from build123d import *

# Parameters (mm, degrees)
F0_W     = 76.2
F0_H     = 50.8
F0_R     = 12.7
F1_DEPTH = 12.7
F2_W     = 6.35
F2_H     = 50.8
F3_DEPTH = 2.54
F5_DEPTH = 50.801
F6_R     = 4.7625
F7_DEPTH = 12.7


with BuildPart() as f1:
    # F0 (on Top) → F1 (new body)
    with BuildSketch(Plane.XY):
        Rectangle(F0_W, F0_H)
        Circle(F0_R, mode=Mode.SUBTRACT)
    extrude(amount=F1_DEPTH)

    # F2 (on face) → F3 (cut)
    with BuildSketch(Plane.XY.offset(12.7)):
        with Locations((-32.385, 0)):
            Rectangle(F2_W, F2_H)
        with BuildLine():
            Line((-5.08, -11.639742), (-5.08, -25.4))
            Line((-5.08, -25.4), (5.08, -25.4))
            Line((5.08, -25.4), (5.08, -11.639742))
            ThreePointArc((5.08, -11.639742), (0, -12.7), (-5.08, -11.639742))
        make_face()
        with BuildLine():
            Line((5.08, 25.4), (-5.08, 25.4))
            Line((-5.08, 25.4), (-5.08, 11.639742))
            ThreePointArc((-5.08, 11.639742), (0, 12.7), (5.08, 11.639742))
            Line((5.08, 11.639742), (5.08, 25.4))
        make_face()
    extrude(amount=-F3_DEPTH, mode=Mode.SUBTRACT)

    # F4 (on face) → F5 (cut, through all)
    with BuildSketch(Plane.XZ.offset(25.4)):
        Polygon((31.75, 12.7), (19.05, 12.7), (16.117061, 7.62), (34.682939, 7.62), align=None)
    extrude(amount=-F5_DEPTH, mode=Mode.SUBTRACT)

    # F6 (on face) → F7 (join)
    with BuildSketch(Plane.YZ.offset(38.1)):
        with Locations((0, 6.35)):
            Circle(F6_R)
    extrude(amount=F7_DEPTH)


solid = f1.part
Verification items for the finished model (mm, model axes). A direction names the side the tool comes from. Give positions to 0.01 mm unless a question says otherwise; leave off trailing zeros. Order: outer loops, then holes, each group sorted by start corner. A loop starts at its lowest first (then second) coordinate and runs counter-clockwise, first axis right, second up. Notation, with made-up numbers: (64, -6) -> (123, -6) arc R19 cw to (123, 6) -> close; hole circle Ø6 at (83.25, 56.25). An arc over 180 degrees is marked (long way). Answer as CSV lines item,"result".
Q1. Release check for a two-part mould opening along X. For faces 4 (the flat face through (38.1, 5, 6)), 5 (the flat face through (-5.08, -18, 11)), 6 (the flat face through (-1, 25.4, 6)) record: +X half, -X half, draft (parallel to the pull), parting line (faces both ways), or undercut.
Solutions:
face 4,"+X half"
face 5,"undercut"
face 6,"draft"
Q2. Sectioned sample at D-D on y = -16. Record the cut outline in (x, z).
Solutions:
outline,"(-38.1, 0) -> (38.1, 0) -> (38.1, 12.7) -> (31.75, 12.7) -> (34.68, 7.62) -> (16.12, 7.62) -> (19.05, 12.7) -> (5.08, 12.7) -> (5.08, 10.16) -> (-5.08, 10.16) -> (-5.08, 12.7) -> (-29.21, 12.7) -> (-29.21, 10.16) -> (-35.56, 10.16) -> (-35.56, 12.7) -> (-38.1, 12.7) -> close"
Q3. Sectioned sample at A-A on y = 0. Record the cut outline in (x, z).
Solutions:
outline,"(-38.1, 0) -> (-12.7, 0) -> (-12.7, 12.7) -> (-29.21, 12.7) -> (-29.21, 10.16) -> (-35.56, 10.16) -> (-35.56, 12.7) -> (-38.1, 12.7) -> close; (12.7, 0) -> (38.1, 0) -> (38.1, 1.59) -> (50.8, 1.59) -> (50.8, 11.11) -> (38.1, 11.11) -> (38.1, 12.7) -> (31.75, 12.7) -> (34.68, 7.62) -> (16.12, 7.62) -> (19.05, 12.7) -> (12.7, 12.7) -> close"
Q4. Depth check by flat-ended pin: pin 1 (2 mm diameter, centred on y = -10.5, z = 11, fed in from +X); pin 2 (1.9 mm diameter, centred on x = -31, y = -10, fed in from +Z). Enter the tip coordinate at first touch or a pass-through.
Solutions:
pin 1,"stops at x = 38.1"
pin 2,"stops at z = 10.16"
Q5. Sectioned sample at C-C on z = 6.35. Record the cut outline in (x, y).
Solutions:
outline,"(-38.1, -25.4) -> (38.1, -25.4) -> (38.1, -4.76) -> (50.8, -4.76) -> (50.8, 4.76) -> (38.1, 4.76) -> (38.1, 25.4) -> (-38.1, 25.4) -> close; hole circle Ø25.4 at (0, 0)"
Q6. Sectioned sample at B-B on x = 0. Record the cut outline in (y, z).
Solutions:
outline,"(-25.4, 0) -> (-12.7, 0) -> (-12.7, 10.16) -> (-25.4, 10.16) -> close; (12.7, 0) -> (25.4, 0) -> (25.4, 10.16) -> (12.7, 10.16) -> close"
Q7. Scan lines: probe 1 along X at (y, z) = (0, 10.25); probe 2 along X at (y, z) = (0, 9); probe 3 along X at (y, z) = (8.5, 8). Record each from-to range of solid material in increasing order.
Solutions:
probe 1,"x = -38.1 to -35.56, -29.21 to -12.7, 12.7 to 17.64, 33.16 to 50.8"
probe 2,"x = -38.1 to -12.7, 12.7 to 16.91, 33.89 to 50.8"
probe 3,"x = -38.1 to -9.44, 9.44 to 16.34, 34.46 to 38.1"
Q8. Access from +Z, -Z, +X, -X, +Y, -Y to the whole of each face (thin tool, end or side, straight path). Record for faces 1 (the flat face through (35, 0, 12.7)), 2 (the flat face through (5.08, 18, 11)), 3 (the flat face through (33.24, -0.36, 10.12)).
Solutions:
face 1,"+Z, +X, -X, +Y, -Y"
face 2,"+Z, +Y, -Y"
face 3,"+Y, -Y"
